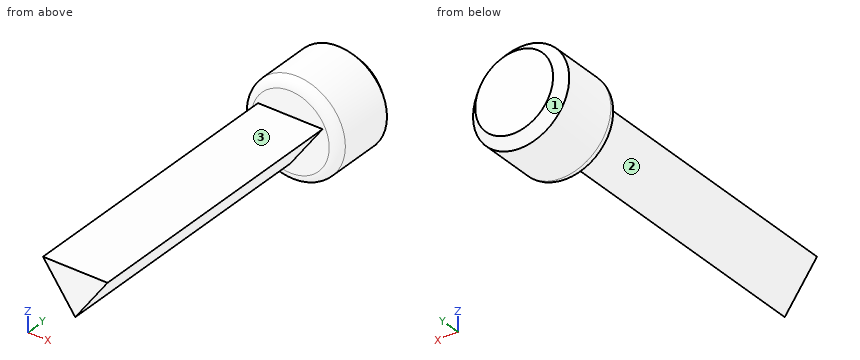
```python
from build123d import *

# Parameters (mm, degrees)
F1_DEPTH = 155
F2_R     = 26.10915
F3_DEPTH = 40
F4_SIZE  = 5
F5_R     = 5


with BuildPart() as f1:
    # F0 (on Front) → F1 (new body)
    with BuildSketch(Plane.XZ):
        Polygon((17.5, 8.122329), (-17.5, 8.122329), (0, -16.244657), align=None)
    extrude(amount=F1_DEPTH)

    # F2 (on Front) → F3 (join)
    with BuildSketch(Plane.XZ):
        Circle(F2_R)
    extrude(amount=-F3_DEPTH)

    # F4
    f4_edges = [f1.edges().sort_by_distance(p)[0] for p in [
        (-26.10915, 40, 0),
    ]]
    chamfer(f4_edges, length=F4_SIZE)

    # F5
    f5_edges = [f1.edges().sort_by_distance(p)[0] for p in [
        (-26.10915, 0, 0),
    ]]
    fillet(f5_edges, radius=F5_R)


solid = f1.part
```
CAD build for the part. Positions are in the model's coordinates, mm. Face numbers are marked on the shaded views. A direction names the side the tool comes from. Coordinates: 2 decimals unless noted, no trailing zeros. Loops run counter-clockwise (first coordinate to the right, second up) from the corner with the lowest first, then second, coordinate; pieces in that order, holes last. Notation, with made-up numbers: (-17.5, -28.75) - (15.5, -28.75) arc R11 cw to (15.5, -8.75) - close; hole circle Ø10 at (21.5, -34.75). An arc over 180 degrees is marked (long way). Return JSON: item names as keys, results as strings.
1. 3-axis set-ups, long thin cutter, end or side, ignore diameter. For the marked faces 1, 2 and 3: which of +Z, -Z, +X, -X, +Y, -Y reach the whole face in a straight line?
Result:
{"face 1": "+Y", "face 2": "-Z, -X, -Y", "face 3": "+Z, +X, -X, -Y"}
2. Band-saw the part on A-A (z = 0). Give the cut face in (x, y), and give its area (3 significant figures).
Result:
{"outline": "(-26.11, 5) arc R5 ccw to (-21.11, 0) - (-11.67, 0) - (-11.67, -155) - (11.67, -155) - (11.67, 0) - (21.11, 0) arc R5 ccw to (26.11, 5) - (26.11, 35) - (21.11, 40) - (-21.11, 40) - (-26.11, 35) - close", "area": "5,670 mm2"}
3. Probe L1, parallel to Y at x = 6.5, z = -8; L2, parallel to X at y = -125, z = 6; L3, parallel to X at y = -109, z = -5.5. List the from-to ranges inside material, lowest first. Write a range as from..to.
Result:
{"L1": "y = 0..40", "L2": "x = -15.98..15.98", "L3": "x = -7.72..7.72"}
4. Drop flat-ended pins along their axis: pin 1 (1 mm diameter, centred on y = 14.5, z = 5.5, fed in from -X); pin 2 (2 mm diameter, centred on y = 9.5, z = 8.5, fed in from +X); pin 3 (8 mm diameter, centred on x = 9, y = -135, fed in from -Z). Give the stop position or say it passes through.
Result:
{"pin 1": "stops at x = -25.63", "pin 2": "stops at x = 25.01", "pin 3": "stops at z = -9.28"}
5. Band-saw the part on B-B (y = -84). Give the cut face in (x, z), and give its area (3 significant figures).
Result:
{"outline": "(-17.5, 8.12) - (0, -16.24) - (17.5, 8.12) - close", "area": "426 mm2"}
